from build123d import *

# Parameters (mm, degrees)
SKETCH1_W               = 14.3002
SKETCH1_H               = 15.875
BOSS_EXTRUDE1_DEPTH     = 10.9728
CUT_EXTRUDE1_DEPTH      = 20.695226989
CUT_EXTRUDE1_DEPTH_BACK = 20.695226989
CUT_EXTRUDE2_DEPTH      = 16.314378084
CUT_EXTRUDE2_DEPTH_BACK = 16.314378084
SKETCH6_W               = 3.646294
SKETCH6_H               = 15.875


with BuildPart() as part:
    # Sketch1 → Boss-Extrude1 (new body)
    with BuildSketch(Plane(origin=(0, 0, 0), x_dir=(1, 0, 0), z_dir=(0, 1, 0))):
        Rectangle(SKETCH1_W, SKETCH1_H)
    extrude(amount=BOSS_EXTRUDE1_DEPTH)

    # Sketch5 → Cut-Extrude1 (cut, two sides: drawn at the far end of the back side and taken through both)
    with BuildSketch(Plane(origin=(7.1501, 0, 0), x_dir=(0, 0, -1), z_dir=(1, 0, 0)).offset(-CUT_EXTRUDE1_DEPTH_BACK)):
        with BuildLine():
            Line((-5.334, 10.9728), (5.334, 10.9728))
            Line((5.334, 10.9728), (5.334, 9.779))
            ThreePointArc((5.334, 9.779), (5.214968196, 9.491631804), (4.9276, 9.3726))
            Line((4.9276, 9.3726), (-4.9276, 9.3726))
            ThreePointArc((-4.9276, 9.3726), (-5.214968196, 9.491631804), (-5.334, 9.779))
            Line((-5.334, 9.779), (-5.334, 10.9728))
        make_face()
    extrude(amount=CUT_EXTRUDE1_DEPTH + CUT_EXTRUDE1_DEPTH_BACK, mode=Mode.SUBTRACT)

    # Sketch3 → Cut-Revolve1 (revolve, cut)
    with BuildSketch(Plane(origin=(0, 0, 0), x_dir=(0, 0, -1), z_dir=(1, 0, 0)), mode=Mode.PRIVATE) as cut_revolve1_sk:
        Polygon((-3.6703, 9.3726), (-3.2639, 8.9662), (-3.2639, 2.2098), (-2.7686, 1.7145), (-2.7686, 0), (-1.27, 0), (-1.27, 9.3726), align=None)
    revolve(cut_revolve1_sk.sketch.rotate(Axis((0, 0, 1.27), (0, 1, 0)), 180), axis=Axis((0, 0, 1.27), (0, 1, 0)), mode=Mode.SUBTRACT)

    # Sketch4 → Cut-Revolve2 (revolve, cut)
    with BuildSketch(Plane(origin=(4.1402, 0, 0), x_dir=(0, 0, -1), z_dir=(1, 0, 0)), mode=Mode.PRIVATE) as cut_revolve2_sk:
        Polygon((2.9972, 10.9728), (2.9972, 0), (4.4972, 0), (4.4972, 8.9662), (4.9036, 9.3726), (4.9036, 10.9728), align=None)
    revolve(cut_revolve2_sk.sketch.rotate(Axis((4.1402, 10.9728, -2.9972), (0, -1, 0)), 180), axis=Axis((4.1402, 10.9728, -2.9972), (0, -1, 0)), mode=Mode.SUBTRACT)

    # Sketch6 → Cut-Extrude2 (cut, two sides: drawn at the far end of the back side and taken through both)
    with BuildSketch(Plane(origin=(0, 10.9728, 0), x_dir=(1, 0, 0), z_dir=(0, 1, 0)).offset(-CUT_EXTRUDE2_DEPTH_BACK)):
        with Locations((-5.326953, 0)):
            Rectangle(SKETCH6_W, SKETCH6_H)
    extrude(amount=CUT_EXTRUDE2_DEPTH + CUT_EXTRUDE2_DEPTH_BACK, mode=Mode.SUBTRACT)


solid = part.part
Geometry check sheet. Reference: the model listing, model coordinates, mm. A direction names the side the tool comes from. Round coordinates to 2 decimals unless told otherwise and drop trailing zeros. Write each loop counter-clockwise with the first axis right and the second up, starting at its lowest first coordinate (ties: lowest second). Pieces come first, ordered by that corner, then holes.
Item 1: Section check B-B (x = 0). Record the boundary of the cut face in (y, z), plus the area to 3 significant figures.
Determined:
outline: (0, -7.94) - (10.97, -7.94) - (10.97, -5.33) - (9.78, -5.33) arc R0.41 cw to (9.37, -4.93) - (9.37, -1.13) - (8.97, -0.72) - (2.21, -0.72) - (1.71, -0.23) - (0, -0.23) - close; (0, 2.77) - (1.71, 2.77) - (2.21, 3.26) - (8.97, 3.26) - (9.37, 3.67) - (9.37, 4.93) arc R0.41 cw to (9.78, 5.33) - (10.97, 5.33) - (10.97, 7.94) - (0, 7.94) - close
area: 122 mm2
Item 2: Access from +Z, -Z, +X, -X, +Y, -Y to the whole of each face (thin tool, end or side, straight path). Record for faces 4 (the face through (2, 10, 5.334)), 5 (the face through (-1.35, 5.54, 2.74)), 6 (the face through (7.15, 5, 0)).
Determined:
face 4: +X, -X, +Y
face 5: +Y
face 6: +Z, -Z, +X, +Y, -Y
Item 3: Section check D-D (z = 4.5). Record the boundary of the cut face in (x, y).
Determined:
outline: (-3.5, 0) - (7.15, 0) - (7.15, 9.37) - (-3.5, 9.37) - close
Item 4: Section check A-A (z = 1.27). Record the boundary of the cut face in (x, y), plus the area to 3 significant figures.
Determined:
outline: (-3.5, 0) - (-1.5, 0) - (-1.5, 1.71) - (-1.99, 2.21) - (-1.99, 8.97) - (-2.4, 9.37) - (-3.5, 9.37) - close; (1.5, 0) - (7.15, 0) - (7.15, 9.37) - (2.4, 9.37) - (1.99, 8.97) - (1.99, 2.21) - (1.5, 1.71) - close
area: 64.3 mm2
Item 5: Material ranges on line 1 along X through (y, z) = (1.15, 1.27); line 2 along X through (y, z) = (6, 1.27); line 3 along Z through (x, y) = (-2.5, 10), recorded low to high.
Determined:
line 1: x = -3.5 to -1.5, 1.5 to 7.15
line 2: x = -3.5 to -1.99, 1.99 to 7.15
line 3: z = -7.94 to -5.33, 5.33 to 7.94
Item 6: Go/stop test with flat-tipped pins: pin 1 Ø4 at (x, z) = (-1.5, 2.5) entering from -Y; pin 2 Ø2.5 at (x, z) = (4.14, -3) entering from -Y; pin 3 Ø5 at (x, z) = (0, 1.27) entering from +Y. Record where each tip stops, or that it passes through.
Determined:
pin 1: stops at y = 0
pin 2: passes through
pin 3: stops at y = 9.37
Item 7: Mould release check, pull along Z, two halves, no side actions. Record for faces 1 (the face through (-3.504, 5, 0)), 2 (the face through (2, 5, -7.938)), 3 (the face through (-0.066, 0.845, 2.767)): +Z half, -Z half, draft (parallel to the pull), parting line (faces both ways), or undercut.
Determined:
face 1: draft
face 2: -Z half
face 3: undercut
Item 8: Section check C-C (y = 5). Record the boundary of the cut face in (x, z), plus the area to 3 significant figures.
Determined:
outline: (-3.5, -7.94) - (7.15, -7.94) - (7.15, 7.94) - (-3.5, 7.94) - close; hole circle Ø3.99 at (0, 1.27); hole circle Ø3 at (4.14, -3)
area: 150 mm2
